CAD build for the part. Positions are in the model's coordinates, mm. A direction names the side the tool comes from. Give positions to 0.01 mm unless a question says otherwise; leave off trailing zeros. Write each loop counter-clockwise with the first axis right and the second up, starting at its lowest first coordinate (ties: lowest second). Pieces come first, ordered by that corner, then holes. Notation, with made-up numbers: M -39,-7.5 L -25,-7.5 A22 cw -25,4.5 Z; hole C -11,13 d11. An arc over 180 degrees is marked long. One line per question, with ' | ' between items. Start each with the question number.
1. Flat gauge pins, fed straight in: pin 1 (1 mm diameter, centred on y = 6.5, z = 2, fed in from -X); pin 2 (2.5 mm diameter, centred on y = 29.5, z = 29.5, fed in from -X). Where does each tip first touch, or does it go through?
2. Wall check: L1, parallel to Y at x = -2.1, z = -29.5; L2, parallel to Y at x = 0.5, z = 29.5. Give the ranges that are in metal, low to high.
3. Pull direction Y, two halves, no side cores. Call faces 1 (the face through (0.4, -8.1, -34.25)), 2 (the face through (0.4, -34.25, -7.1)), 3 (the face through (-1.972, 25.865, 26.067)), 4 (the face through (-1.972, -26.966, -26.736)): released by +Y, released by -Y, zero draft, split by the parting line, or undercut.
4. Cut at D-D, the plane y = -2. Write the cut outline in (x, z), then the cut area to 3 significant figures.
5. Cut at C-C, the plane x = -1.6. Write the cut outline in (y, z), then the cut area to 3 significant figures.
6. Which spindle directions (+Z, -Z, +X, -X, +Y, -Y) get a long thin tool onto all of the face, cutting with end or side? Do faces 5 (the face through (-1.972, -25.865, -26.067)), 6 (the face through (0.4, 34.25, 7.1)). Say none if no direction does.
7. Cut at A-A, the plane z = -29.5. Write the cut outline in (x, y).
Autodesk Inventor part; units mm, degrees
ref_plane "YZ Plane" through (0, 0, 0) normal (1, 0, 0) x (0, 1, 0)
ref_plane "XZ Plane" through (0, 0, 0) normal (0, 1, 0) x (-1, 0, 0)
ref_plane "XY Plane" through (0, 0, 0) normal (0, 0, 1) x (1, 0, 0)
sketch "Sketch1" plane through (0, 0, 0) normal (1, 0, 0) x (0, 1, 0)
  line L0 (34.5, 34.5) -> (-34.5, 34.5)
  line L1 (-34.5, 34.5) -> (-34.5, -34.5)
  line L2 (-34.5, -34.5) -> (34.5, -34.5)
  line L3 (34.5, -34.5) -> (34.5, 34.5)
  line L4 (34.5, 34.5) -> (-34.5, -34.5) construction
  line L5 (-34.5, 34.5) -> (34.5, -34.5) construction
  point P0 (0, 0)
  dimension "d0" = 69
  dimension "d1" = 69
extrude "Extrusion1" add sketch "Sketch1" along normal blind 2
sketch "Sketch2" plane through (0, 0, 0) normal (-1, 0, 0) x (0, 0, 1)
  circle A0 centre (29.5, 29.5) radius 3.75
  circle A1 centre (29.5, 29.5) radius 5
  line L0 (-34.5, 34.5) -> (34.5, 34.5)
  line L1 (34.5, 34.5) -> (34.5, -34.5)
  circle A2 centre (29.5, 29.5) radius 2.15
  point P0 (0, 0)
  point P1 (34.5, 29.5)
  point P2 (29.5, 34.5)
  dimension "d4" = 7.5
  dimension "d5" = 10
  dimension "d6" = 5
  dimension "d7" = 5
  dimension "d10" = 4.3
extrude "Extrusion2" add sketch "Sketch2" along normal blind 4 contours A1 | A1 L0 L1
extrude "Extrusion3" cut sketch "Sketch2" against normal blind 4 contours A2
pattern_circular "Circular Pattern1" count 2 over 360 about axis through (-10, 0, 0) along (1, 0, 0) of "Extrusion2", "Extrusion3"
sketch "Sketch3" plane through (2, 0, 0) normal (1, 0, 0) x (0, 0, -1)
  circle A0 centre (29.5, -29.5) radius 2.15
  circle A1 centre (-29.5, 29.5) radius 2.15
  line L0 (-34.5, -34.5) -> (34.5, -34.5)
  line L1 (34.5, -34.5) -> (34.5, 34.5)
  line L2 (34.5, 34.5) -> (-34.5, 34.5)
  line L3 (-34.5, 34.5) -> (-34.5, -34.5)
  line L4 (-34.25, -34.25) -> (34.25, -34.25)
  line L5 (34.25, -34.25) -> (34.25, 34.25)
  line L6 (34.25, 34.25) -> (-34.25, 34.25)
  line L7 (-34.25, 34.25) -> (-34.25, -34.25)
  line L8 (-34.25, -34.25) -> (34.25, 34.25) construction
  line L9 (34.25, -34.25) -> (-34.25, 34.25) construction
  point P0 (0, 0)
  dimension "d16" = 0.25
  dimension "d17" = 0.25
extrude "Extrusion4" cut sketch "Sketch3" against normal through all contours L3 L2 L1 L0
properties part number "pokrywa_obudowa"
Here are the results:
1) pin 1: x = 0 | pin 2: through
2) L1: -34.25 to -33.25, -25.75 to -24.5 | L2: -34.25 to 27.35, 31.65 to 34.25
3) face 1: zero draft | face 2: released by -Y | face 3: split by the parting line | face 4: undercut
4) outline: M 0,-34.25 L 2,-34.25 L 2,34.25 L 0,34.25 Z | area: 137 mm^2
5) outline: M -34.25,-34.25 L -27.94,-34.25 A5 ccw long -34.25,-27.94 Z; M 27.94,34.25 A5 ccw long 34.25,27.94 L 34.25,34.25 Z; hole C -29.5,-29.5 d7.5; hole C 29.5,29.5 d7.5 | area: 73.5 mm^2
6) face 5: -X | face 6: +Z, -Z, +X, -X, +Y
7) outline: M -4,-34.25 L 2,-34.25 L 2,-31.65 L 0,-31.65 L 0,-33.25 L -4,-33.25 Z; M -4,-25.75 L 0,-25.75 L 0,-27.35 L 2,-27.35 L 2,34.25 L 0,34.25 L 0,-24.5 L -4,-24.5 Z
